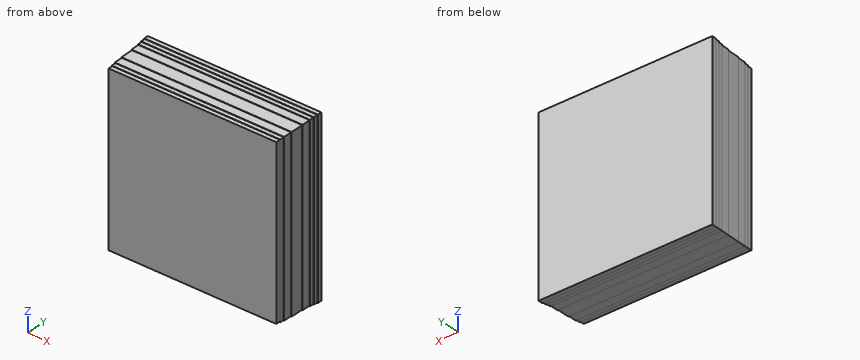
```python
from build123d import *

# Parameters (mm, degrees)
F0_W      = 40
F0_H      = 40
F1_DEPTH  = 1
F2_W      = 39.8
F2_H      = 39.8
F3_DEPTH  = 2
F4_W      = 39.6
F4_H      = 39.6
F5_DEPTH  = 3
F6_W      = 39.4
F6_H      = 39.4
F7_DEPTH  = 1
F8_W      = 39.4
F8_H      = 39.4
F9_DEPTH  = 1
F10_W     = 39.2
F10_H     = 39.2
F11_DEPTH = 1
F12_W     = 39
F12_H     = 39
F13_DEPTH = 1
F14_W     = 40.2
F14_H     = 40.2
F15_DEPTH = 1
F16_W     = 40.4
F16_H     = 40.4
F17_DEPTH = 1


with BuildPart() as f1:
    # F0 (on Front) → F1 (new body)
    with BuildSketch(Plane.XZ):
        Rectangle(F0_W, F0_H)
    extrude(amount=F1_DEPTH)

    # F2 (on face) → F3 (join)
    with BuildSketch(Plane.XZ.offset(1)):
        Rectangle(F2_W, F2_H)
    extrude(amount=F3_DEPTH)

    # F4 (on face) → F5 (join)
    with BuildSketch(Plane.XZ.offset(3)):
        Rectangle(F4_W, F4_H)
    extrude(amount=F5_DEPTH)



with BuildPart() as f7:
    # F6 (on face) → F7 (new body)
    with BuildSketch(Plane.XZ.offset(7)):
        Rectangle(F6_W, F6_H)
    extrude(amount=F7_DEPTH)


with BuildPart() as f1_1:
    add(f1.part)

    add(f7.part)  # F9 merges F7
    # F8 (on face) → F9 (join)
    with BuildSketch(Plane.XZ.offset(6)):
        Rectangle(F8_W, F8_H)
    extrude(amount=F9_DEPTH)

    # F10 (on face) → F11 (join)
    with BuildSketch(Plane.XZ.offset(8)):
        Rectangle(F10_W, F10_H)
    extrude(amount=F11_DEPTH)

    # F12 (on face) → F13 (join)
    with BuildSketch(Plane.XZ.offset(9)):
        Rectangle(F12_W, F12_H)
    extrude(amount=F13_DEPTH)

    # F14 (on face) → F15 (join)
    with BuildSketch(Plane(origin=(0, 0, 0), x_dir=(-1, 0, 0), z_dir=(0, 1, 0))):
        Rectangle(F14_W, F14_H)
    extrude(amount=F15_DEPTH)

    # F16 (on face) → F17 (join)
    with BuildSketch(Plane(origin=(0, 1, 0), x_dir=(-1, 0, 0), z_dir=(0, 1, 0))):
        Rectangle(F16_W, F16_H)
    extrude(amount=F17_DEPTH)


solid = f1_1.part
```
The listing builds one solid part. Answer for the finished solid, in the listing's coordinates (mm). Give positions to 0.01 mm unless a question says otherwise; leave off trailing zeros. Order: outer loops, then holes, each group sorted by start corner. A loop starts at its lowest first (then second) coordinate and runs counter-clockwise, first axis right, second up. Notation, with made-up numbers: M 28,72 L 52,72 A20 ccw 52,82 Z; hole C -31,-21.5 d11. An arc over 180 degrees is marked long. Put each result on its own line as item: value. Start each with the question number.
Item 1: The part is cut by section C-C, the plane y = -2.25. Determine the outline of the cut face in (x, z).
Item 2: Find the intervals of material crossed by line 1 along X through (y, z) = (-7.75, 1); line 2 along X through (y, z) = (-8.5, 12.5); line 3 along Z through (x, y) = (-13, -2.75), in increasing order.
Item 3: Flat-ended cylindrical pins translate along their axes: P1, Ø3, axis at x = -3, y = -8, coming from the -Z side; P2, Ø0.6, axis at y = -7.5, z = -9.5, coming from the -X side; P3, Ø1.5, axis at y = -4, z = 5, coming from the -X side. Find the tip coordinate at first contact, or state that the pin passes through.
Item 4: The part is cut by section D-D, the plane y = -4.75. Determine the outline of the cut face in (x, z).
Answer key:
1. outline: M -19.9,-19.9 L 19.9,-19.9 L 19.9,19.9 L -19.9,19.9 Z
2. line 1: x = -19.7 to 19.7
2. line 2: x = -19.6 to 19.6
2. line 3: z = -19.9 to 19.9
3. P1: stops at z = -19.7
3. P2: stops at x = -19.7
3. P3: stops at x = -19.8
4. outline: M -19.8,-19.8 L 19.8,-19.8 L 19.8,19.8 L -19.8,19.8 Z
